```python
from build123d import *

# Parameters (mm, degrees)
F0_W     = 192.9788589478
F0_H     = 182.3403686285
F1_DEPTH = 12.7
F4_R     = 12.69999


# Not quite as in the source:
# - a fillet or chamfer is up to 0.001 mm smaller than in the source, because OpenCascade refuses the exact size
# - the program builds the solid bodies; features that only make, move or delete a surface that nothing else refers to are left out


with BuildPart() as f1:
    # F0 (on Top) → F1 (new body)
    with BuildSketch(Plane.XY):
        Rectangle(F0_W, F0_H)
    extrude(amount=F1_DEPTH)

    # F4 (radius 12.7 in the source; OpenCascade refuses exactly that, so slightly less here)
    f4_edges = [f1.edges().sort_by_distance(p)[0] for p in [
        (0, 91.170184, 12.7),
    ]]
    fillet(f4_edges, radius=F4_R)


solid = f1.part
```
The model under review builds one solid part; all positions refer to its coordinate system, in mm. Give positions to 0.01 mm unless a question says otherwise; leave off trailing zeros. Order: outer loops, then holes, each group sorted by start corner. A loop starts at its lowest first (then second) coordinate and runs counter-clockwise, first axis right, second up. Notation, with made-up numbers: (79, 73) - (95, 73) arc R20 ccw to (95, 86) - close; hole circle Ø8 at (7, -8.75). An arc over 180 degrees is marked (long way). Use CSV: the item, a comma, the result in double quotes. Start each with the question number.
Q1. Clearance check with flat-ended pins moving along their axes: pin 1 Ø3 at (x, z) = (70.5, 10.5) entering from +Y; pin 2 Ø4 at (x, z) = (26.5, 6.5) entering from +Y. State where each tip first meets the part, or that it passes through.
Q2. To check wall thickness, follow line 1 along Y through (x, z) = (-51, 1); line 2 along Y through (x, z) = (-32, 11). State the ranges of each line that lie inside material, in increasing order. Write a range as [from, to].
Q3. We need section A-A, the plane z = 8.75. Write out the cut boundary in (x, y).
Outcome:
1,pin 1,"stops at y = 87.43"
1,pin 2,"stops at y = 90.35"
2,line 1,"y = [-91.17, 91.13]"
2,line 2,"y = [-91.17, 84.82]"
3,outline,"(-96.49, -91.17) - (96.49, -91.17) - (96.49, 87.67) - (-96.49, 87.67) - close"
